Geometry check sheet. Reference: the model listing, model coordinates, mm. A direction names the side the tool comes from. Coordinates: 2 decimals unless noted, no trailing zeros. Write each loop counter-clockwise with the first axis right and the second up, starting at its lowest first coordinate (ties: lowest second). Pieces come first, ordered by that corner, then holes.
from build123d import *

# Parameters (mm, degrees)
FILLET1_R = 0.2


with BuildPart() as part:
    # Sketch1 → Revolve1 (revolve)
    with BuildSketch(Plane(origin=(0, 0, 0), x_dir=(0, 0, -1), z_dir=(1, 0, 0))):
        Polygon((0, 0), (0, 3.265), (4.63, 3.265), (4.63, 3.96), (39.19, 3.96), (39.19, 3.485), (51, 3.485), (51, 0), align=None)
    revolve(axis=Axis((0, 0, 22.591484059), (0, 0, -1)))

    # Fillet1
    fillet1_edges = [part.edges().sort_by_distance(p)[0] for p in [
        (0, -3.265, 0),
    ]]
    fillet(fillet1_edges, radius=FILLET1_R)


solid = part.part
1. Thickness scan on line 1 along Z through (x, y) = (-1, 3.5); line 2 along X through (y, z) = (0.25, -43.5); line 3 along Y through (x, z) = (-0.25, -35). Record the ranges inside material, lowest first.
Computed values:
line 1: z = -39.19 to -4.63
line 2: x = -3.48 to 3.48
line 3: y = -3.95 to 3.95
2. Sectioned sample at D-D, the plane z = -14.5. Record the boundary of the cut face in (x, y).
Computed values:
outline: circle Ø7.92 at (0, 0)
3. Sectioned sample at C-C, the plane z = -42. Record the boundary of the cut face in (x, y) (3 decimals), and give its area (3 significant figures).
Computed values:
outline: circle Ø6.97 at (0, 0)
area: 38.2 mm2
4. Sectioned sample at A-A, the plane y = 0. Record the boundary of the cut face in (x, z) (3 decimals), and give its area (3 significant figures).
Computed values:
outline: (-3.96, -39.19) - (-3.485, -39.19) - (-3.485, -51) - (3.485, -51) - (3.485, -39.19) - (3.96, -39.19) - (3.96, -4.63) - (3.265, -4.63) - (3.265, -0.2) arc R0.2 ccw to (3.065, 0) - (-3.065, 0) arc R0.2 ccw to (-3.265, -0.2) - (-3.265, -4.63) - (-3.96, -4.63) - close
area: 386 mm2
5. Access from +Z, -Z, +X, -X, +Y, -Y to the whole of each face (thin tool, end or side, straight path). Record for faces 1 (the flat face through (0, 0, 0)), 2 (the cylindrical face through (-3.09, 1.61, -45.18)), 3 (the flat face through (3, 2, -4.63)).
Computed values:
face 1: +Z, +X, -X, +Y, -Y
face 2: -Z
face 3: +Z
6. Gauge pin test, flat ends, axial feed: pin 1 Ø1.5 at (y, z) = (-3, -11.5) entering from +X; pin 2 Ø2 at (x, z) = (3, -36.5) entering from +Y. Record the tip position at first contact, or that the pin passes through.
Computed values:
pin 1: stops at x = 3.26
pin 2: stops at y = 3.42
